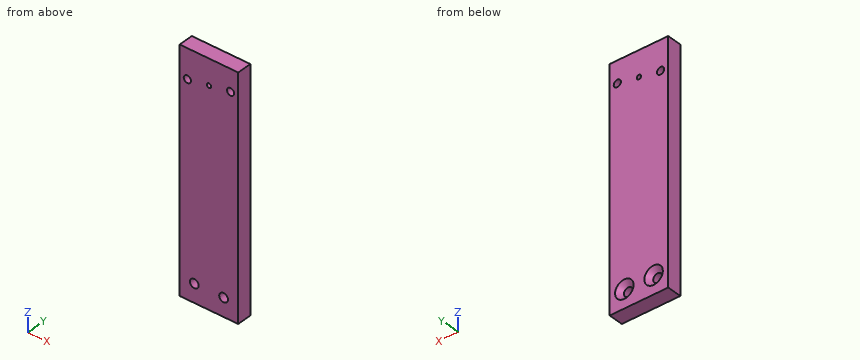
Autodesk Inventor part; units mm, degrees
ref_plane "YZ Plane" through (0, 0, 0) normal (1, 0, 0) x (0, 1, 0)
ref_plane "XZ Plane" through (0, 0, 0) normal (0, 1, 0) x (-1, 0, 0)
ref_plane "XY Plane" through (0, 0, 0) normal (0, 0, 1) x (1, 0, 0)
sketch "Sketch1" plane through (0, 0, 0) normal (0, 0, 1) x (1, 0, 0)
  line L0 (-20, 5) -> (20, 5)
  line L1 (20, 5) -> (20, -5)
  line L2 (20, -5) -> (-20, -5)
  line L3 (-20, -5) -> (-20, 5)
  line L4 (-20, 5) -> (20, -5) construction
  line L5 (20, 5) -> (-20, -5) construction
  point P0 (0, 0)
extrude "Extrusion1" add sketch "Sketch1" along normal mid plane 162.5
sketch "Sketch4" plane through (-20, 5, 81.25) normal (0, 1, 0) x (1, 0, 0)
  line L0 (0, 162.5) -> (40, 162.5)
  point P0 (20, 81.25)
  point P1 (10, 150)
  point P2 (30, 150)
  dimension "d28" = 10
  dimension "d29" = 20
  dimension "d30" = 12.5
hole "Hole3" at (-10, 5, -68.75) at (10, 5, -68.75) direction (0, -1, 0) diameter 6 depth 10.4 countersink diameter 12.6 countersink angle 90
sketch "Sketch5" plane through (-20, 5, 81.25) normal (0, 1, 0) x (1, 0, 0)
  circle A0 centre (30, 150) radius 6.3
  point P0 (20, 81.25)
  point P1 (20, 17.5)
  dimension "d38" = 132.5
hole "Hole4" at (0, 5, 63.75) direction (0, -1, 0) diameter 3 depth 10.4
sketch "Sketch6" plane through (-20, 5, 81.25) normal (0, 1, 0) x (1, 0, 0)
  circle A0 centre (20, 17.5) radius 1.5
  line L0 (20, 17.5) -> (3, 17.5) construction
  line L1 (5.23, 20.1043) -> (20, 17.5) construction
  line L2 (20, 17.5) -> (34.77, 14.8957) construction
  point P0 (20, 81.25)
  dimension "d46" = 10
  dimension "d47" = 10
  dimension "d48" = 14.77
  dimension "d49" = 14.77
hole "Hole5" at (-14.77, 5, 61.1457) at (14.77, 5, 66.3543) direction (0, -1, 0) diameter 4.917 depth 17.1
equation "\"d49\" = d48"
properties part number "Support Beam" material "Brass, Soft Yellow"
Source: CAD feature listing. Evaluate the final solid. Frame: model axes, mm. Coordinates: 2 decimals unless noted, no trailing zeros. Order: outer loops, then holes, each group sorted by start corner. A loop starts at its lowest first (then second) coordinate and runs counter-clockwise, first axis right, second up. Notation, with made-up numbers: (51.5, 28) - (82.5, 28) arc R30 cw to (82.5, 65) - close; hole circle Ø3 at (-21.5, 38.25). An arc over 180 degrees is marked (long way). One line per item, written item: value.
1) Cut plane B-B on x = 0. Output: boundary loops of the cut face in (y, z), plus the area to 4 significant figures.
Computed values:
outline: (-5, -81.25) - (5, -81.25) - (5, 62.25) - (-5, 62.25) - close; (-5, 65.25) - (5, 65.25) - (5, 81.25) - (-5, 81.25) - close
area: 1,595 mm^2
2) Ray query, line 1 (X direction, y = 3.75, z = 61); line 2 (Z direction, x = -10, y = -3); line 3 (Z direction, x = 14.77, y = 2.75). Return the intervals inside material, ascending. Write a range as [from, to].
Computed values:
line 1: x = [-20, -17.22], [-12.32, 20]
line 2: z = [-81.25, -71.75], [-65.75, 81.25]
line 3: z = [-81.25, 63.9], [68.81, 81.25]
3) Contact query for flat-ended pins moving along their axis: pin 1 (5.5 mm diameter, centred on x = 10, z = -68.75, fed in from +Y); pin 2 (7 mm diameter, centred on x = -10, z = -68.75, fed in from +Y). Output: stop coordinate, or through.
Computed values:
pin 1: passes through
pin 2: stops at y = 2.2
4) Cut plane C-C on x = -10. Output: boundary loops of the cut face in (y, z).
Computed values:
outline: (-5, -81.25) - (5, -81.25) - (5, -75.05) - (1.7, -71.75) - (-5, -71.75) - close; (-5, -65.75) - (1.7, -65.75) - (5, -62.45) - (5, 81.25) - (-5, 81.25) - close
5) Cut plane A-A on y = -2.25. Output: boundary loops of the cut face in (x, z).
Computed values:
outline: (-20, -81.25) - (20, -81.25) - (20, 81.25) - (-20, 81.25) - close; hole circle Ø4.92 at (-14.77, 61.15); hole circle Ø6 at (-10, -68.75); hole circle Ø3 at (0, 63.75); hole circle Ø6 at (10, -68.75); hole circle Ø4.92 at (14.77, 66.35)
